Input: part model. Units: mm. Frame: model coordinates. Give positions to 0.01 mm unless a question says otherwise; leave off trailing zeros. Order: outer loops, then holes, each group sorted by start corner. A loop starts at its lowest first (then second) coordinate and runs counter-clockwise, first axis right, second up. Notation, with made-up numbers: M 44.5,70.5 L 68.5,70.5 A19 ccw 68.5,81.5 Z; hole C -24,41.5 d2. An arc over 180 degrees is marked long. Use a Markdown table: item, result.
from build123d import *

# Parameters (mm, degrees)
ESQUISSE1_R        = 1.05
ESQUISSE1_R_2      = 3
BOSS_EXTRU_1_DEPTH = 2


with BuildPart() as part:
    # Esquisse1 → Boss.-Extru.1 (new body)
    with BuildSketch(Plane.XY):
        with BuildLine():
            ThreePointArc((-5.945158342, 6.756855207), (-9, 0), (-5.945158342, -6.756855207))
            Line((-5.945158342, -6.756855207), (0, -7.5))
            ThreePointArc((0, -7.5), (7.5, 0), (0, 7.5))
            Line((0, 7.5), (-5.945158342, 6.756855207))
        make_face()
        with Locations((-4.772970773, 4.772970773)):
            Circle(ESQUISSE1_R, mode=Mode.SUBTRACT)
        with Locations((-4.772970773, -4.772970773)):
            Circle(ESQUISSE1_R, mode=Mode.SUBTRACT)
        Circle(ESQUISSE1_R_2, mode=Mode.SUBTRACT)
        with Locations((5.5, 0)):
            Circle(ESQUISSE1_R, mode=Mode.SUBTRACT)
    extrude(amount=BOSS_EXTRU_1_DEPTH)


solid = part.part
1) Cut plane D-D on x = 5. Return loops of the section in (y, z), and give its area (3 significant figures).
Response values:
| item | result |
|---|---|
| outline | M -5.59,0 L -0.92,0 L -0.92,2 L -5.59,2 Z; M 0.92,0 L 5.59,0 L 5.59,2 L 0.92,2 Z |
| area | 18.7 mm² |
2) Material intervals for line 1 (X direction, y = 0.5, z = 1); line 2 (Y direction, x = -4, z = 1.3); line 3 (Y direction, x = -1, z = 1.8) (3 decimals), sorted ascending. Write a range as from..to.
Response values:
| item | result |
|---|---|
| line 1 | x = -8.99..-2.96, 2.96..4.58, 6.42..7.48 |
| line 2 | y = -7..-5.48, -4.06..4.06, 5.48..7 |
| line 3 | y = -7.375..-2.828, 2.828..7.375 |
3) Cut plane A-A on y = 0. Return loops of the section in (x, z), and give its area (3 significant figures).
Response values:
| item | result |
|---|---|
| outline | M -9,0 L -3,0 L -3,2 L -9,2 Z; M 3,0 L 4.45,0 L 4.45,2 L 3,2 Z; M 6.55,0 L 7.5,0 L 7.5,2 L 6.55,2 Z |
| area | 16.8 mm² |
4) Mould query, pull axis X, two halves, no side actions, for faces 1 (the face through (4.45, 0.05, 0.99)), 2 (the face through (7.5, -0.16, 0.99)), 3 (the face through (-9, 0, 1)), 4 (the face through (-5.82, 4.82, 0.99)). Classes: released by +X, released by -X, zero draft, split by the parting line, or undercut.
Response values:
| item | result |
|---|---|
| face 1 | undercut |
| face 2 | released by +X |
| face 3 | released by -X |
| face 4 | undercut |
5) First-contact query: pin 1 Ø1 at (y, z) = (-3.5, 1.5) entering from -X; pin 2 Ø1 at (y, z) = (-3.5, 1) entering from +X; pin 3 Ø1 at (y, z) = (-5, 1.5) entering from +X. Flat tips, straight axial feed; report the tip coordinate or a pass-through.
Response values:
| item | result |
|---|---|
| pin 1 | stops at x = -8.49 |
| pin 2 | stops at x = 6.87 |
| pin 3 | stops at x = 6 |
6) Cut plane C-C on z = 0.3. Return loops of the section in (x, y).
Response values:
| item | result |
|---|---|
| outline | M -5.95,-6.76 L 0,-7.5 A7.5 ccw 0,7.5 L -5.95,6.76 A9 ccw Z; hole C -4.77,-4.77 d2.1; hole C -4.77,4.77 d2.1; hole C 0,0 d6; hole C 5.5,0 d2.1 |
7) Cut plane B-B on y = 2. Return loops of the section in (x, z), and give its area (3 significant figures).
Response values:
| item | result |
|---|---|
| outline | M -8.77,0 L -2.24,0 L -2.24,2 L -8.77,2 Z; M 2.24,0 L 7.23,0 L 7.23,2 L 2.24,2 Z |
| area | 23.1 mm² |
